Geometry check sheet. Reference: drawing and pictorial views, mm from the part's lowest x, y, z. A direction names the side the tool comes from. Round coordinates to 2 decimals unless told otherwise and drop trailing zeros. Loops run counter-clockwise (first coordinate to the right, second up) from the corner with the lowest first, then second, coordinate; pieces in that order, holes last. Notation, with made-up numbers: (59.5, -39) -> (102.5, -39) arc R22 cw to (102.5, -33) -> close; hole circle Ø4 at (-6, 46.5). An arc over 180 degrees is marked (long way). Use one line per item in the form item = value.
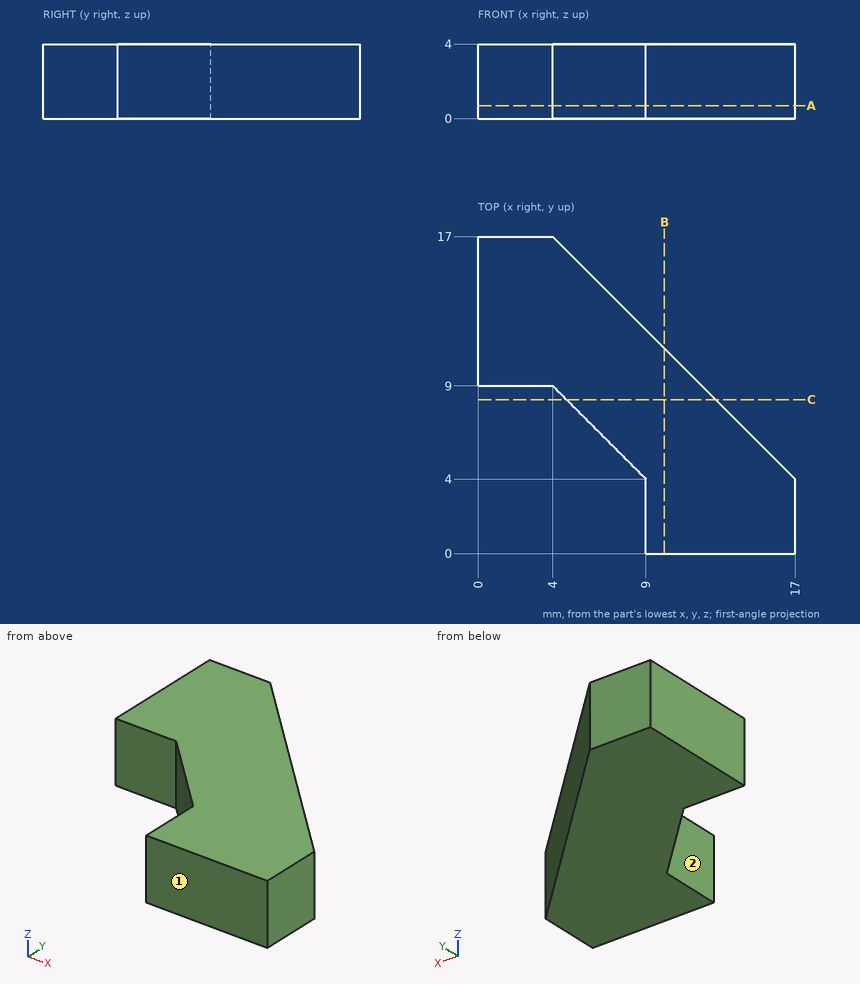
1. Gauge pin test, flat end, axial feed: pin 1 (2 mm diameter, centred on y = 1.5, z = 1.5, fed in from -X). Record the tip position at first contact, or that the pin passes through.
Return value:
pin_1 = 9
2. Section check C-C (y = 8.25). Record the boundary of the cut face in (x, z), then the cut area to 3 significant figures.
Return value:
outline = (4.75, 0) -> (12.75, 0) -> (12.75, 4) -> (4.75, 4) -> close
area = 32.0 mm2
3. Tool access check on the marked faces 1 and 2. Record the directions out of +Z, -Z, +X, -X, +Y, -Y that give a thin tool (end or side, any length) a straight path to the whole face; none if there is none.
Return value:
face_1 = +Z, -Z, +X, -X, -Y
face_2 = +Z, -Z, -X, -Y
4. Section check B-B (x = 10). Record the boundary of the cut face in (y, z).
Return value:
outline = (0, 0) -> (11, 0) -> (11, 4) -> (0, 4) -> close
5. Section check A-A (z = 0.7). Record the boundary of the cut face in (x, y), then the cut area to 3 significant figures.
Return value:
outline = (0, 9) -> (4, 9) -> (9, 4) -> (9, 0) -> (17, 0) -> (17, 4) -> (4, 17) -> (0, 17) -> close
area = 136 mm2
6. Material ranges on line 1 along Y through (x, z) = (2.75, 3.5); line 2 along Y through (x, z) = (14.5, 2.4), recorded low to high.
Return value:
line_1 = 9 to 17
line_2 = 0 to 6.5
